from build123d import *

# Parameters (mm, degrees)
ESQUISSE1_R                  = 35
ESQUISSE1_R_2                = 25
BOSS_EXTRU_1_DEPTH           = 2
BOSS_EXTRU_2_START           = 26
ESQUISSE2_R                  = 1.8
BOSS_EXTRU_2_DEPTH           = 8
R_P_TITION_CIRCULAIRE1_COUNT = 20


with BuildPart() as part:
    # Esquisse1 → Boss.-Extru.1 (new body)
    with BuildSketch(Plane.XY):
        Circle(ESQUISSE1_R)
        Circle(ESQUISSE1_R_2, mode=Mode.SUBTRACT)
    extrude(amount=BOSS_EXTRU_1_DEPTH)

    # Esquisse2 → Boss.-Extru.2 (add)
    with BuildSketch(Plane(origin=(0, 0, 0), x_dir=(1, 0, 0), z_dir=(0, 1, 0)).offset(BOSS_EXTRU_2_START)):
        with Locations((0, -1)):
            Circle(ESQUISSE2_R)
    boss_extru_2 = extrude(amount=BOSS_EXTRU_2_DEPTH)

    # Répétition circulaire1: Boss.-Extru.2 ×20 about axis
    r_p_tition_circulaire1_axis = Axis((0, 0, 0), (0, 0, 1))
    for i in range(1, R_P_TITION_CIRCULAIRE1_COUNT):
        add(boss_extru_2.rotate(r_p_tition_circulaire1_axis, i * 360 / R_P_TITION_CIRCULAIRE1_COUNT))


solid = part.part
Can you work these out from the model? Positions are in its coordinate system, mm. A direction names the side the tool comes from. Give positions to 0.01 mm unless a question says otherwise; leave off trailing zeros. Order: outer loops, then holes, each group sorted by start corner. A loop starts at its lowest first (then second) coordinate and runs counter-clockwise, first axis right, second up. Notation, with made-up numbers: M -32,11 L 3,11 A24 cw 3,35 Z; hole C 26.25,-37.5 d7. An arc over 180 degrees is marked long. One line per item, written item: value.
Item 1: If we section it at C-C on z = 1.45: Write out the boundary of the cut face in (x, y), and give its area (3 significant figures).
Verdict:
outline: C 0,0 d70; hole C 0,0 d50
area: 1,880 mm2
Item 2: If we section it at A-A on x = 0: Write out the boundary of the cut face in (y, z).
Verdict:
outline: M -35,0 L -34,0 L -34,-0.8 L -26,-0.8 L -26,0 L -25,0 L -25,2 L -26,2 L -26,2.8 L -34,2.8 L -34,2 L -35,2 Z; M 25,0 L 26,0 L 26,-0.8 L 34,-0.8 L 34,0 L 35,0 L 35,2 L 34,2 L 34,2.8 L 26,2.8 L 26,2 L 25,2 Z
Item 3: For pin 1 (0.6 mm diameter, centred on x = 0.5, z = -0.5, fed in from -Y); pin 2 (0.6 mm diameter, centred on y = 0.5, z = -0.5, fed in from +X); pin 3 (0.6 mm diameter, centred on x = -0.5, z = 2, fed in from -Y), each with a flat end and sliding along its axis, tell me the tip position at first contact or that it passes through.
Verdict:
pin 1: y = -34
pin 2: x = 34
pin 3: y = -35
Item 4: For faces 5 (the face through (21.047, -15.265, 2.306)), 6 (the face through (-27.519, 19.968, 2.306)), 7 (the face through (-15.3, 21.02, -0.32)), 8 (the face through (-27.494, -20.002, 2.306)), 9 (the face through (0, 29.9, 2.8)), which set-ups out of +Z, -Z, +X, -X, +Y, -Y let a thin tool reach every point of the face, with its end or its side?
Verdict:
face 5: +Z
face 6: +Z, -X, +Y
face 7: -Z
face 8: +Z, -X, -Y
face 9: +Z, +Y, -Y
Item 5: Please list where these lines run through material, in increasing order: line 1 (Y direction, x = 0, z = 0.5); line 2 (X direction, y = 0, z = -0.45); line 3 (Y direction, x = 8, z = 1.2).
Verdict:
line 1: -35 to -25, 25 to 35
line 2: -34 to -26, 26 to 34
line 3: -34.07 to -23.69, 23.69 to 34.07
Item 6: If we mould it in two halves opening along X, with no side actions, what happens to faces 1 (the face through (29.9, 0, -0.8)), 2 (the face through (-20.002, 27.494, 2.306)), 3 (the face through (-9.2, -28.5, 2.8)), 4 (the face through (19.968, 27.519, 2.306))? For each: pulls with the +X half, pulls with the -X half, needs draft (parallel to the pull), parting line crosses it, or undercut.
Verdict:
face 1: needs draft
face 2: pulls with the -X half
face 3: undercut
face 4: pulls with the +X half
